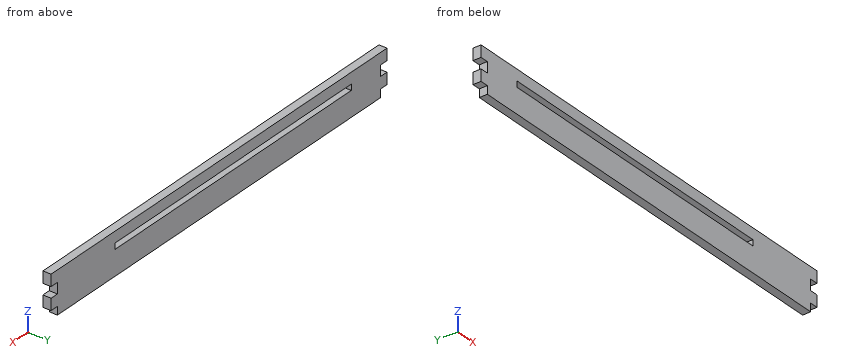
```python
from build123d import *

# Parameters (mm, degrees)
F0_W     = 254
F0_H     = 24.7625
F1_DEPTH = 4.7625
F2_W     = 4.7625
F2_H     = 6.35
F3_DEPTH = 25.4
F4_W     = 4.7625
F4_H     = 4.7625
F5_DEPTH = 25.4
F6_W     = 5.5
F6_H     = 3.5
F6_W_2   = 2.5
F6_W_3   = 3
F7_DEPTH = 25.4


with BuildPart() as f1:
    # F0 (on Front) → F1 (new body)
    with BuildSketch(Plane.XZ):
        Rectangle(F0_W, F0_H)
    extrude(amount=F1_DEPTH)

    # F2 (on face) → F3 (cut)
    with BuildSketch(Plane.XZ.offset(4.7625)):
        with Locations((-124.61875, 2.38125)):
            Rectangle(F2_W, F2_H)
        with Locations((124.61875, 2.38125)):
            Rectangle(F2_W, F2_H)
    extrude(amount=-F3_DEPTH, mode=Mode.SUBTRACT)

    # F4 (on face) → F5 (cut)
    with BuildSketch(Plane.XZ.offset(4.7625)):
        with Locations((124.61875, -10)):
            Rectangle(F4_W, F4_H)
        with Locations((-124.61875, -10)):
            Rectangle(F4_W, F4_H)
    extrude(amount=-F5_DEPTH, mode=Mode.SUBTRACT)

    # F6 (on face) → F7 (cut)
    with BuildSketch(Plane.XZ.offset(4.7625)):
        with Locations((-97.250009, 4.13125)):
            Rectangle(F6_W, F6_H)
        with Locations((-93.250009, 4.13125)):
            Rectangle(F6_W_2, F6_H)
        with Locations((-90.500009, 4.13125)):
            Rectangle(F6_W_3, F6_H)
        with Locations((-87.750009, 4.13125)):
            Rectangle(F6_W_2, F6_H)
        with Locations((-85.000009, 4.13125)):
            Rectangle(F6_W_3, F6_H)
        with Locations((-82.250009, 4.13125)):
            Rectangle(F6_W_2, F6_H)
        with Locations((-79.500009, 4.13125)):
            Rectangle(F6_W_3, F6_H)
        with Locations((-76.750009, 4.13125)):
            Rectangle(F6_W_2, F6_H)
        with Locations((-74.000009, 4.13125)):
            Rectangle(F6_W_3, F6_H)
        with Locations((-71.250009, 4.13125)):
            Rectangle(F6_W_2, F6_H)
        with Locations((-68.500009, 4.13125)):
            Rectangle(F6_W_3, F6_H)
        with Locations((-65.750009, 4.13125)):
            Rectangle(F6_W_2, F6_H)
        with Locations((-63.000009, 4.13125)):
            Rectangle(F6_W_3, F6_H)
        with Locations((-60.250009, 4.13125)):
            Rectangle(F6_W_2, F6_H)
        with Locations((-57.500009, 4.13125)):
            Rectangle(F6_W_3, F6_H)
        with Locations((-54.750009, 4.13125)):
            Rectangle(F6_W_2, F6_H)
        with Locations((-52.000009, 4.13125)):
            Rectangle(F6_W_3, F6_H)
        with Locations((-49.250009, 4.13125)):
            Rectangle(F6_W_2, F6_H)
        with Locations((-46.500009, 4.13125)):
            Rectangle(F6_W_3, F6_H)
        with Locations((-43.750009, 4.13125)):
            Rectangle(F6_W_2, F6_H)
        with Locations((-41.000009, 4.13125)):
            Rectangle(F6_W_3, F6_H)
        with Locations((-38.250009, 4.13125)):
            Rectangle(F6_W_2, F6_H)
        with Locations((-35.500009, 4.13125)):
            Rectangle(F6_W_3, F6_H)
        with Locations((-32.750009, 4.13125)):
            Rectangle(F6_W_2, F6_H)
        with Locations((-30.000009, 4.13125)):
            Rectangle(F6_W_3, F6_H)
        with Locations((-27.250009, 4.13125)):
            Rectangle(F6_W_2, F6_H)
        with Locations((-24.500009, 4.13125)):
            Rectangle(F6_W_3, F6_H)
        with Locations((-21.750009, 4.13125)):
            Rectangle(F6_W_2, F6_H)
        with Locations((-19.000009, 4.13125)):
            Rectangle(F6_W_3, F6_H)
        with Locations((-16.250009, 4.13125)):
            Rectangle(F6_W_2, F6_H)
        with Locations((-13.500009, 4.13125)):
            Rectangle(F6_W_3, F6_H)
        with Locations((-10.750009, 4.13125)):
            Rectangle(F6_W_2, F6_H)
        with Locations((-8.000009, 4.13125)):
            Rectangle(F6_W_3, F6_H)
        with Locations((-5.250009, 4.13125)):
            Rectangle(F6_W_2, F6_H)
        with Locations((-2.500009, 4.13125)):
            Rectangle(F6_W_3, F6_H)
        with Locations((0.249991, 4.13125)):
            Rectangle(F6_W_2, F6_H)
        with Locations((2.999991, 4.13125)):
            Rectangle(F6_W_3, F6_H)
        with Locations((5.749991, 4.13125)):
            Rectangle(F6_W_2, F6_H)
        with Locations((8.499991, 4.13125)):
            Rectangle(F6_W_3, F6_H)
        with Locations((11.249991, 4.13125)):
            Rectangle(F6_W_2, F6_H)
        with Locations((13.999991, 4.13125)):
            Rectangle(F6_W_3, F6_H)
        with Locations((16.749991, 4.13125)):
            Rectangle(F6_W_2, F6_H)
        with Locations((19.499991, 4.13125)):
            Rectangle(F6_W_3, F6_H)
        with Locations((22.249991, 4.13125)):
            Rectangle(F6_W_2, F6_H)
        with Locations((24.999991, 4.13125)):
            Rectangle(F6_W_3, F6_H)
        with Locations((27.749991, 4.13125)):
            Rectangle(F6_W_2, F6_H)
        with Locations((30.499991, 4.13125)):
            Rectangle(F6_W_3, F6_H)
        with Locations((33.249991, 4.13125)):
            Rectangle(F6_W_2, F6_H)
        with Locations((35.999991, 4.13125)):
            Rectangle(F6_W_3, F6_H)
        with Locations((38.749991, 4.13125)):
            Rectangle(F6_W_2, F6_H)
        with Locations((41.499991, 4.13125)):
            Rectangle(F6_W_3, F6_H)
        with Locations((44.249991, 4.13125)):
            Rectangle(F6_W_2, F6_H)
        with Locations((46.999991, 4.13125)):
            Rectangle(F6_W_3, F6_H)
        with Locations((49.749991, 4.13125)):
            Rectangle(F6_W_2, F6_H)
        with Locations((52.499991, 4.13125)):
            Rectangle(F6_W_3, F6_H)
        with Locations((55.249991, 4.13125)):
            Rectangle(F6_W_2, F6_H)
        with Locations((57.999991, 4.13125)):
            Rectangle(F6_W_3, F6_H)
        with Locations((60.749991, 4.13125)):
            Rectangle(F6_W_2, F6_H)
        with Locations((63.499991, 4.13125)):
            Rectangle(F6_W_3, F6_H)
        with Locations((66.249991, 4.13125)):
            Rectangle(F6_W_2, F6_H)
        with Locations((68.999991, 4.13125)):
            Rectangle(F6_W_3, F6_H)
        with Locations((71.749991, 4.13125)):
            Rectangle(F6_W_2, F6_H)
        with Locations((75.749991, 4.13125)):
            Rectangle(F6_W, F6_H)
    extrude(amount=-F7_DEPTH, mode=Mode.SUBTRACT)


solid = f1.part
```
The listing builds one solid part. Answer for the finished solid, in the listing's coordinates (mm). Coordinates: 2 decimals unless noted, no trailing zeros. Write each loop counter-clockwise with the first axis right and the second up, starting at its lowest first coordinate (ties: lowest second). Pieces come first, ordered by that corner, then holes.
Q1. Given P1, Ø2.5, axis at x = -124.5, y = -2, coming from the -Z side; P2, Ø2.5, axis at y = -2, z = 4, coming from the +X side; P3, Ø1.8, axis at y = -2.5, z = 4, coming from the -X side, each flat-ended and moving along its own axis, determine where each tip first touches the part or whether it passes through.
Returned:
P1: stops at z = -7.62
P2: stops at x = 122.24
P3: stops at x = -122.24
Q2. Section B-B, the plane x = 8 is taken. Write down the section's boundary in (y, z), then the cut area to 3 significant figures.
Returned:
outline: (-4.76, -12.38) - (0, -12.38) - (0, 2.38) - (-4.76, 2.38) - close; (-4.76, 5.88) - (0, 5.88) - (0, 12.38) - (-4.76, 12.38) - close
area: 101 mm2
Q3. Section C-C, the plane z = -9.75 is taken. Write down the section's boundary in (x, y), then the cut area to 3 significant figures.
Returned:
outline: (-122.24, -4.76) - (122.24, -4.76) - (122.24, 0) - (-122.24, 0) - close
area: 1,160 mm2
Q4. Find the intervals of material crossed by line 1 along X through (y, z) = (-2.7, 4.75); line 2 along Z through (x, y) = (-44, -3.15); line 3 along X through (y, z) = (-1.9, 5.75), in increasing order.
Returned:
line 1: x = -122.24 to -100, 78.5 to 122.24
line 2: z = -12.38 to 2.38, 5.88 to 12.38
line 3: x = -127 to -100, 78.5 to 127
Q5. Section A-A, the plane y = -3 is taken. Write down the section's boundary in (x, z), then the cut area to 3 significant figures.
Returned:
outline: (-127, -7.62) - (-122.24, -7.62) - (-122.24, -12.38) - (122.24, -12.38) - (122.24, -7.62) - (127, -7.62) - (127, -0.79) - (122.24, -0.79) - (122.24, 5.56) - (127, 5.56) - (127, 12.38) - (-127, 12.38) - (-127, 5.56) - (-122.24, 5.56) - (-122.24, -0.79) - (-127, -0.79) - close; hole (-100, 2.38) - (78.5, 2.38) - (78.5, 5.88) - (-100, 5.88) - close
area: 5,560 mm2
